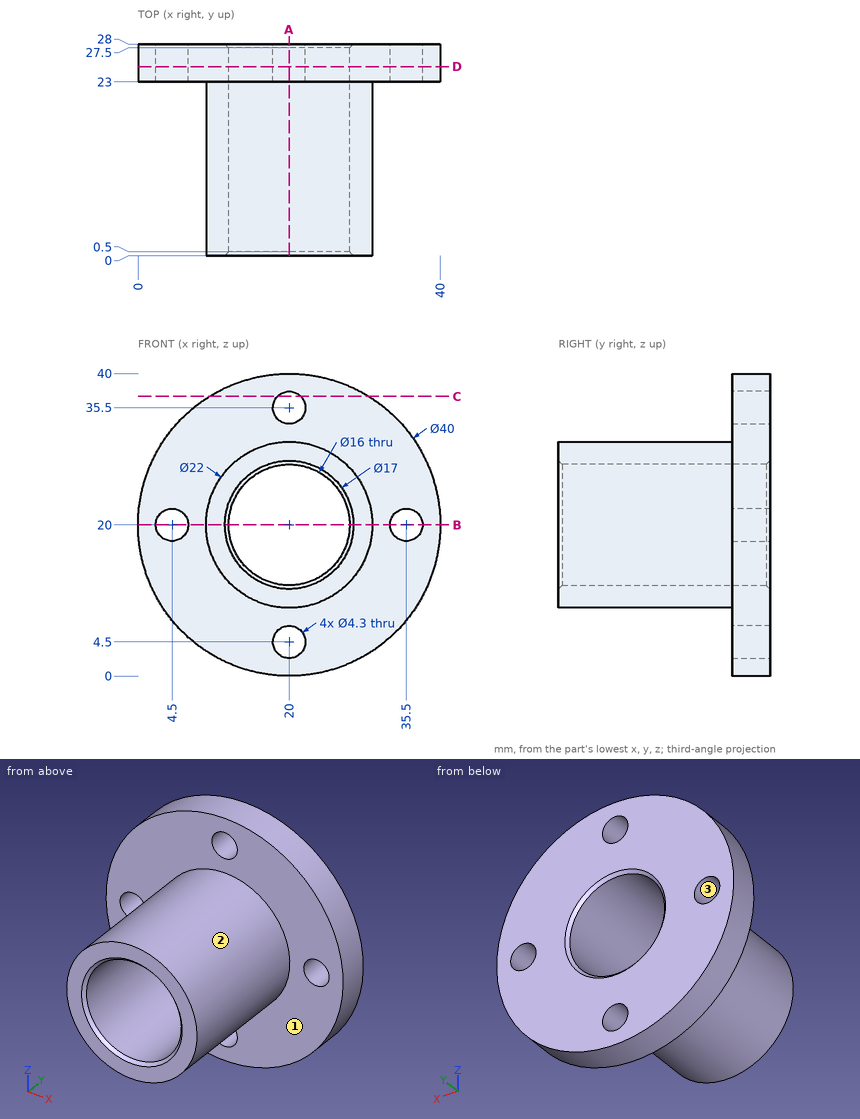
Answer from the drawing. Dimensions are ordinates in mm from the lowest x, y and z of the part. Give positions to 0.01 mm unless a question says otherwise; leave off trailing zeros. Order: outer loops, then holes, each group sorted by start corner. A loop starts at its lowest first (then second) coordinate and runs counter-clockwise, first axis right, second up. Notation, with made-up numbers: (-6.5, 48.25) - (42.5, 48.25) arc R11 ccw to (42.5, 61.25) - close; hole circle Ø2 at (-0.5, -30.5). An arc over 180 degrees is marked (long way). Use one line per item in the form item = value.
1) The mould has two halves that part along X. Classify the marked faces 1, 2 and 3: released by +X, released by -X, zero draft, split by the parting line, or undercut.
Verdict:
face_1 = zero draft
face_2 = split by the parting line
face_3 = undercut
2) Find section D-D on y = 25. Determine the outline of the cut face in (x, z).
Verdict:
outline = circle Ø40 at (20, 20); hole circle Ø4.3 at (4.5, 20); hole circle Ø16 at (20, 20); hole circle Ø4.3 at (20, 4.5); hole circle Ø4.3 at (20, 35.5); hole circle Ø4.3 at (35.5, 20)
3) Find section C-C on z = 37. Determine the outline of the cut face in (x, y).
Verdict:
outline = (9.46, 23) - (18.46, 23) - (18.46, 28) - (9.46, 28) - close; (21.54, 23) - (30.54, 23) - (30.54, 28) - (21.54, 28) - close
4) Find section A-A on x = 20. Determine the outline of the cut face in (y, z), and give its area (4 significant figures).
Verdict:
outline = (0, 9) - (23, 9) - (23, 6.65) - (28, 6.65) - (28, 11.5) - (27.5, 12) - (0.5, 12) - (0, 11.5) - close; (0, 28.5) - (0.5, 28) - (27.5, 28) - (28, 28.5) - (28, 33.35) - (23, 33.35) - (23, 31) - (0, 31) - close; (23, 0) - (28, 0) - (28, 2.35) - (23, 2.35) - close; (23, 37.65) - (28, 37.65) - (28, 40) - (23, 40) - close
area = 214.5 mm^2
5) Each of these flat-tipped pins is pushed along its axis until it touches: pin 1 (1 mm diameter, centred on x = 30.5, y = 20, fed in from -Z); pin 2 (2.5 mm diameter, centred on x = 20, z = 4.5, fed in from +Y); pin 3 (5 mm diameter, centred on y = 19, z = 17, fed in from -X); pin 4 (5.5 mm diameter, centred on x = 35.5, z = 20, fed in from -Y). Where does it stop, or does it pass through?
Verdict:
pin_1 = 15.42
pin_2 = through
pin_3 = 9.01
pin_4 = 23
6) Consider probe 1 along X at (y, z) = (27.05, 20); probe 2 along X at (y, z) = (12, 20); probe 3 along Y at (x, z) = (16.5, 33). Determine where each line is inside the solid, lowest interval first. Write a range as [from, to].
Verdict:
probe_1 = [0, 2.35], [6.65, 12], [28, 33.35], [37.65, 40]
probe_2 = [9, 12], [28, 31]
probe_3 = [23, 28]
7) Find section B-B on z = 20. Determine the outline of the cut face in (x, y).
Verdict:
outline = (0, 23) - (2.35, 23) - (2.35, 28) - (0, 28) - close; (6.65, 23) - (9, 23) - (9, 0) - (11.5, 0) - (12, 0.5) - (12, 27.5) - (11.5, 28) - (6.65, 28) - close; (28, 0.5) - (28.5, 0) - (31, 0) - (31, 23) - (33.35, 23) - (33.35, 28) - (28.5, 28) - (28, 27.5) - close; (37.65, 23) - (40, 23) - (40, 28) - (37.65, 28) - close
